Design review of the part built by this model. Coordinates are the model's own, in mm. Face numbers are marked on the shaded views. Give positions to 0.01 mm unless a question says otherwise; leave off trailing zeros. Loops run counter-clockwise (first coordinate to the right, second up) from the corner with the lowest first, then second, coordinate; pieces in that order, holes last.
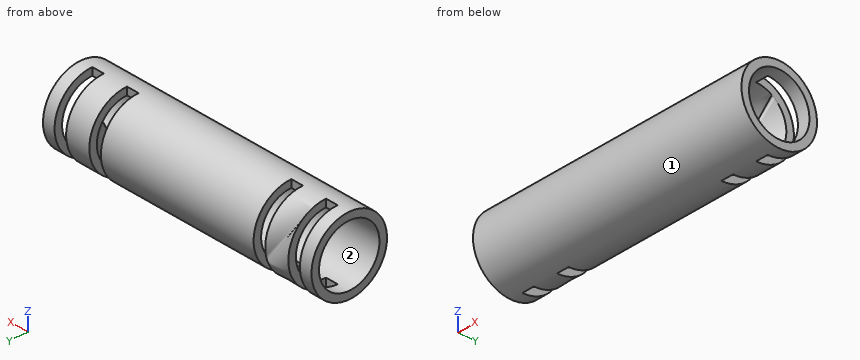
from build123d import *

# Parameters (mm, degrees)
SKETCH2_R           = 7.5
SKETCH2_R_2         = 6
BOSS_EXTRUDE1_DEPTH = 29
CUT_EXTRUDE1_REACH  = 32.879
SKETCH4_W           = 2.5
SKETCH4_H           = 15


with BuildPart() as part:
    # Sketch2 → Boss-Extrude1 (new, symmetric)
    with BuildSketch(Plane(origin=(0, 0, 0), x_dir=(0, 0, -1), z_dir=(1, 0, 0))):
        with Locations(Location((0, 0, 0), (0, 0, 180))):
            Circle(SKETCH2_R)
        with Locations(Location((0, 0, 0), (0, 0, 180))):
            Circle(SKETCH2_R_2, mode=Mode.SUBTRACT)
    extrude(amount=BOSS_EXTRUDE1_DEPTH, both=True)

    # Sketch4 → Cut-Extrude1 (cut, up to next)
    with BuildSketch(Plane(origin=(0, 0, 0), x_dir=(1, 0, 0), z_dir=(0, 1, 0)), mode=Mode.PRIVATE) as cut_extrude1_sk1:
        with Locations((25.25, 0)):
            Rectangle(SKETCH4_W, SKETCH4_H)
    cut_extrude1_tool1 = extrude(cut_extrude1_sk1.sketch, amount=CUT_EXTRUDE1_REACH, mode=Mode.PRIVATE) & part.part
    # Sketch4 → Cut-Extrude1 (cut, up to next)
    with BuildSketch(Plane(origin=(0, 0, 0), x_dir=(1, 0, 0), z_dir=(0, 1, 0)), mode=Mode.PRIVATE) as cut_extrude1_sk2:
        with Locations((17.75, 0)):
            Rectangle(SKETCH4_W, SKETCH4_H)
    cut_extrude1_tool2 = extrude(cut_extrude1_sk2.sketch, amount=CUT_EXTRUDE1_REACH, mode=Mode.PRIVATE) & part.part
    # Sketch4 → Cut-Extrude1 (cut, up to next)
    with BuildSketch(Plane(origin=(0, 0, 0), x_dir=(1, 0, 0), z_dir=(0, 1, 0)), mode=Mode.PRIVATE) as cut_extrude1_sk3:
        with Locations((-17.75, 0)):
            Rectangle(SKETCH4_W, SKETCH4_H)
    cut_extrude1_tool3 = extrude(cut_extrude1_sk3.sketch, amount=CUT_EXTRUDE1_REACH, mode=Mode.PRIVATE) & part.part
    # Sketch4 → Cut-Extrude1 (cut, up to next)
    with BuildSketch(Plane(origin=(0, 0, 0), x_dir=(1, 0, 0), z_dir=(0, 1, 0)), mode=Mode.PRIVATE) as cut_extrude1_sk4:
        with Locations((-25.25, 0)):
            Rectangle(SKETCH4_W, SKETCH4_H)
    cut_extrude1_tool4 = extrude(cut_extrude1_sk4.sketch, amount=CUT_EXTRUDE1_REACH, mode=Mode.PRIVATE) & part.part
    add(cut_extrude1_tool1.solids().sort_by_distance((25.25, 0, 0))[0], mode=Mode.SUBTRACT)
    add(cut_extrude1_tool2.solids().sort_by_distance((17.75, 0, 0))[0], mode=Mode.SUBTRACT)
    add(cut_extrude1_tool3.solids().sort_by_distance((-17.75, 0, 0))[0], mode=Mode.SUBTRACT)
    add(cut_extrude1_tool4.solids().sort_by_distance((-25.25, 0, 0))[0], mode=Mode.SUBTRACT)


solid = part.part
Q1. Take a section at D-D (z = -3.5). Give the boundary of the cut face in (x, y), plus the area to 3 significant figures.
Results:
outline: (-29, -6.63) - (29, -6.63) - (29, -4.87) - (-29, -4.87) - close; (-29, 4.87) - (-26.5, 4.87) - (-26.5, 6.63) - (-29, 6.63) - close; (-24, 4.87) - (-19, 4.87) - (-19, 6.63) - (-24, 6.63) - close; (-16.5, 4.87) - (16.5, 4.87) - (16.5, 6.63) - (-16.5, 6.63) - close; (19, 4.87) - (24, 4.87) - (24, 6.63) - (19, 6.63) - close; (26.5, 4.87) - (29, 4.87) - (29, 6.63) - (26.5, 6.63) - close
area: 187 mm2
Q2. Draft analysis for pull direction Y (two halves, no side actions). For the marked faces 1 and 2, state which applies: pulls with the +Y half, pulls with the -Y half, needs draft (parallel to the pull), parting line crosses it, or undercut.
Results:
face 1: parting line crosses it
face 2: undercut
Q3. Take a section at A-A (z = 0). Give the boundary of the cut face in (x, y), plus the area to 3 significant figures.
Results:
outline: (-29, -7.5) - (29, -7.5) - (29, -6) - (-29, -6) - close; (-29, 6) - (-26.5, 6) - (-26.5, 7.5) - (-29, 7.5) - close; (-24, 6) - (-19, 6) - (-19, 7.5) - (-24, 7.5) - close; (-16.5, 6) - (16.5, 6) - (16.5, 7.5) - (-16.5, 7.5) - close; (19, 6) - (24, 6) - (24, 7.5) - (19, 7.5) - close; (26.5, 6) - (29, 6) - (29, 7.5) - (26.5, 7.5) - close
area: 159 mm2
Q4. Take a section at B-B (y = -0.5). Give the boundary of the cut face in (x, z), plus the area to 3 significant figures.
Results:
outline: (-29, -7.48) - (29, -7.48) - (29, -5.98) - (-29, -5.98) - close; (-29, 5.98) - (29, 5.98) - (29, 7.48) - (-29, 7.48) - close
area: 174 mm2
Q5. Insertion check: pin 1 (1.2 mm diameter, centred on x = -18, z = 6.5, fed in from +Y); pin 2 (1.5 mm diameter, centred on x = -13, z = 3.5, fed in from -Y); pin 3 (3 mm diameter, centred on x = 19, y = -5.5, fed in from -Z). Each pin has a flat end and moves straight along its axis. Give the tip position at first contact, or say it passes through.
Results:
pin 1: stops at y = 0
pin 2: stops at y = -6.98
pin 3: stops at z = -6.34
Q6. Wall thickness on line 1 (Z direction, x = 14.5, y = -0.25); line 2 (Y direction, x = 7.5, z = 0); line 3 (X direction, y = 5.25, z = -5.25): over which ranges is each line inside the solid? List them lowest first.
Results:
line 1: z = -7.5 to -5.99, 5.99 to 7.5
line 2: y = -7.5 to -6, 6 to 7.5
line 3: x = -29 to -26.5, -24 to -19, -16.5 to 16.5, 19 to 24, 26.5 to 29
Q7. Take a section at C-C (x = -10). Give the boundary of the cut face in (y, z), plus the area to 3 significant figures.
Results:
outline: circle Ø15 at (0, 0); hole circle Ø12 at (0, 0)
area: 63.6 mm2
